Verification items for the finished model (mm, model axes). A direction names the side the tool comes from. Round coordinates to 2 decimals unless told otherwise and drop trailing zeros. Order: outer loops, then holes, each group sorted by start corner. A loop starts at its lowest first (then second) coordinate and runs counter-clockwise, first axis right, second up. Notation, with made-up numbers: (-2, -14) -> (32, -14) arc R7 cw to (32, -7) -> close; hole circle Ø3 at (60.5, 33). An arc over 180 degrees is marked (long way). Put each result on its own line as item: value.
from build123d import *

# Parameters (mm, degrees)
BOSS_EXTRUDE1_DEPTH = 7.9375
SKETCH3_R           = 5.207
CUT_EXTRUDE1_DEPTH  = 3.96875
SKETCH4_R           = 1.2065
BOSS_EXTRUDE2_DEPTH = 8.89
SKETCH5_W           = 5.08
SKETCH5_H           = 15.875
BOSS_EXTRUDE3_DEPTH = 16.764
SKETCH6_R           = 1.143
CUT_EXTRUDE2_DEPTH  = 12.7


with BuildPart() as part:
    # Sketch1 → Boss-Extrude1 (new, symmetric)
    with BuildSketch(Plane(origin=(0, 0, 0), x_dir=(1, 0, 0), z_dir=(0, 1, 0))):
        Polygon((-2.757708096, -19.86108723), (1.211041904, -19.86108723), (1.211041904, 41.25766277), (58.361041904, 41.25766277), (58.361041904, 45.22641277), (6.27967861, 45.22641277), (-2.757708096, 45.22641277), align=None)
    extrude(amount=BOSS_EXTRUDE1_DEPTH, both=True)

    # Sketch3 → Cut-Extrude1 (cut)
    with BuildSketch(Plane.ZY.offset(2.757708096)):
        with Locations((-12.566559842, 0)):
            Circle(SKETCH3_R)
    extrude(amount=-CUT_EXTRUDE1_DEPTH, mode=Mode.SUBTRACT)

    # Sketch4 → Boss-Extrude2 (add)
    with BuildSketch(Plane(origin=(0, 0, -45.22641277), x_dir=(-1, 0, 0), z_dir=(0, 0, -1))):
        with Locations(Location((-22.007291904, 0, 0), (0, 0, 180))):
            Circle(SKETCH4_R)
    extrude(amount=BOSS_EXTRUDE2_DEPTH)

    # Sketch5 → Boss-Extrude3 (add)
    with BuildSketch(Plane.ZY.offset(2.757708096)):
        with Locations((-20.948559842, 0)):
            Rectangle(SKETCH5_W, SKETCH5_H)
        with Locations((15.373440158, 0)):
            Rectangle(SKETCH5_W, SKETCH5_H)
    extrude(amount=BOSS_EXTRUDE3_DEPTH)

    # Sketch6 → Cut-Extrude2 (cut)
    with BuildSketch(Plane.ZY.offset(19.521708096)):
        with Locations((14.855640158, 0)):
            Circle(SKETCH6_R)
        with Locations((-21.034559842, 0)):
            Circle(SKETCH6_R)
    extrude(amount=-CUT_EXTRUDE2_DEPTH, mode=Mode.SUBTRACT)


solid = part.part
Item 1: Gauge pin test, flat ends, axial feed: pin 1 Ø5 at (x, y) = (-11.5, -0.5) entering from +Z; pin 2 Ø10 at (x, z) = (5.5, -1.5) entering from +Y; pin 3 Ø0.7 at (y, z) = (0, -21) entering from -X; pin 4 Ø3.5 at (y, z) = (0, 14.86) entering from +X. Record the tip position at first contact, or that the pin passes through.
Check sheet entries:
pin 1: stops at z = 17.91
pin 2: stops at y = 7.94
pin 3: stops at x = -6.82
pin 4: stops at x = 1.21
Item 2: Tool access check on faces 4 (the flat face through (-6.822, 0, -21)), 5 (the flat face through (-11, 0, -18.409)), 6 (the flat face through (29, 0, -41.258)), 7 (the flat face through (-11, 0, -23.489)), 8 (the flat face through (-11, 0, 17.913)). Record the directions out of +Z, -Z, +X, -X, +Y, -Y that give a thin tool (end or side, any length) a straight path to the whole face; none if there is none.
Check sheet entries:
face 4: -X
face 5: -X, +Y, -Y
face 6: +Z, +X, +Y, -Y
face 7: -Z, -X, +Y, -Y
face 8: +Z, -X, +Y, -Y
Item 3: Release check for a two-part mould opening along Y. For faces 1 (the flat face through (-1, -7.938, -22)), 2 (the flat face through (1.211, -5, -10)), 3 (the flat face through (-6.822, 0, 15)) record: +Y half, -Y half, draft (parallel to the pull), parting line (faces both ways), or undercut.
Check sheet entries:
face 1: -Y half
face 2: draft
face 3: undercut
Item 4: Section check C-C on z = 4.5. Record the boundary of the cut face in (x, y).
Check sheet entries:
outline: (-2.76, -7.94) -> (1.21, -7.94) -> (1.21, 7.94) -> (-2.76, 7.94) -> close
Item 5: Section check B-B on z = -14. Record the boundary of the cut face in (x, y).
Check sheet entries:
outline: (-2.76, -7.94) -> (1.21, -7.94) -> (1.21, -5.01) -> (-2.76, -5.01) -> close; (-2.76, 5.01) -> (1.21, 5.01) -> (1.21, 7.94) -> (-2.76, 7.94) -> close
Item 6: Material ranges on L1, parallel to Z at x = -6, y = -5; L2, parallel to Z at x = 15.5, y = -4.5; L3, parallel to X at y = 6, z = 3, recorded low to high. Write a range as [from, to].
Check sheet entries:
L1: z = [-23.49, -18.41], [12.83, 17.91]
L2: z = [-45.23, -41.26]
L3: x = [-2.76, 1.21]
